```python
from build123d import *

# Parameters (mm, degrees)
PAD002_DEPTH    = 12.7
SKETCH003_W     = 152.4
SKETCH003_H     = 25.4
SKETCH003_R     = 6.35
PAD003_DEPTH    = 12.7
SKETCH006_R     = 3.175
POCKET001_DEPTH = 6.35
FILLET_R        = 12.446
SKETCH_W        = 76.2
SKETCH_H        = 50.8
SKETCH_W_2      = 73.2
SKETCH_H_2      = 47.8
PAD_DEPTH       = 1042.67
SKETCH001_W     = 76.2
SKETCH001_H     = 50.8
SKETCH001_W_2   = 73.2
SKETCH001_H_2   = 47.8
PAD001_DEPTH    = 914.4
SKETCH004_R     = 3.96875
POCKET_DEPTH    = 6.35
PAD004_DEPTH    = 1016


with BuildPart() as frameupright:
    # Sketch002 → Pad002 (new body, symmetric)
    with BuildSketch(Plane.YZ):
        Polygon((38.1, 878.1034), (38.1, 25.4), (-38.1, 25.4), (-38.1, 746.121128), align=None)
    extrude(amount=PAD002_DEPTH, both=True)

    # Sketch003 (on Face4 of Pad002) → Pad003 (join)
    with BuildSketch(Plane(origin=(0, -351.654926, 203.028066), x_dir=(0, -0.5, -0.866025), z_dir=(0, -0.866025, 0.5))):
        with Locations((-703.309852, 0)):
            Rectangle(SKETCH003_W, SKETCH003_H)
        with Locations((-754.109852, 0)):
            Circle(SKETCH003_R, mode=Mode.SUBTRACT)
        with Locations((-652.509852, 0)):
            Circle(SKETCH003_R, mode=Mode.SUBTRACT)
    extrude(amount=PAD003_DEPTH)

    # Sketch006 (on Face1 of Pad003) → Pocket001 (cut)
    with BuildSketch(Plane.ZX.offset(38.1)):
        with Locations((714.375, -0.082469)):
            Circle(SKETCH006_R)
    extrude(amount=-POCKET001_DEPTH, mode=Mode.SUBTRACT)

    # Fillet
    fillet_edges = [frameupright.edges().sort_by_distance(p)[0] for p in [
        (0, 27.101477, 884.4534),
    ]]
    fillet(fillet_edges, radius=FILLET_R)


with BuildPart() as frameupright_1:
    # Body001 placement: moved
    add(frameupright.part.moved(Location((-1029.1, 0, 0))))


with BuildPart() as frameupright001:
    # Link base: copy of FrameUpright
    add(frameupright_1.part)


with BuildPart() as frameupright001_1:
    # Link placement: moved
    add(frameupright001.part.moved(Location((2057.8, 0, 0))))


with BuildPart() as fusion:
    # Sketch → Pad (new body, symmetric)
    with BuildSketch(Plane.YZ):
        Rectangle(SKETCH_W, SKETCH_H)
        Rectangle(SKETCH_W_2, SKETCH_H_2, mode=Mode.SUBTRACT)
    extrude(amount=PAD_DEPTH, both=True)

    # Sketch001 (on DatumPlane) → Pad001 (join)
    with BuildSketch(Plane(origin=(-1079.5, -609.6, 0), x_dir=(1, 0, 0), z_dir=(0, -1, 0))):
        Rectangle(SKETCH001_W, SKETCH001_H)
        Rectangle(SKETCH001_W_2, SKETCH001_H_2, mode=Mode.SUBTRACT)
        with Locations((2159, 0)):
            Rectangle(SKETCH001_W, SKETCH001_H)
        with Locations((2159, 0)):
            Rectangle(SKETCH001_W_2, SKETCH001_H_2, mode=Mode.SUBTRACT)
    extrude(amount=-PAD001_DEPTH)

    # Sketch004 (on Face12 of Pad001) → Pocket (cut)
    with BuildSketch(Plane.YX.offset(25.4)):
        with Locations((-588.9498, -1057.275)):
            Circle(SKETCH004_R)
        with Locations((-512.7498, -1057.275)):
            Circle(SKETCH004_R)
        with Locations((-588.9498, -1101.725)):
            Circle(SKETCH004_R)
        with Locations((-512.7498, -1101.725)):
            Circle(SKETCH004_R)
        with Locations((207.9498, -1057.275)):
            Circle(SKETCH004_R)
        with Locations((207.9498, -1101.725)):
            Circle(SKETCH004_R)
        with Locations((284.1498, -1057.275)):
            Circle(SKETCH004_R)
        with Locations((284.1498, -1101.725)):
            Circle(SKETCH004_R)
    pocket = extrude(amount=-POCKET_DEPTH, mode=Mode.SUBTRACT)

    # Mirrored: Pocket across Sketch004 H_Axis
    add(pocket.mirror(Plane(origin=(0, 0, -25.4), x_dir=(0, 0, -1), z_dir=(1, 0, 0))), mode=Mode.SUBTRACT)

    # Sketch005 → Pad004 (join, symmetric)
    with BuildSketch(Plane.YZ):
        Polygon((30.1625, 38.1), (33.3375, 38.1), (33.3375, 25.4), (20.6375, 25.4), (20.6375, 28.575), (30.1625, 28.575), align=None)
    extrude(amount=PAD004_DEPTH, both=True)

    # Fusion: union FrameUpright, FrameUpright001
    add(frameupright_1.part)
    add(frameupright001_1.part)


solid = fusion.part
```
Part model, mm, in its own coordinate system. A direction names the side the tool comes from. Coordinates: 2 decimals unless noted, no trailing zeros. Order: outer loops, then holes, each group sorted by start corner. A loop starts at its lowest first (then second) coordinate and runs counter-clockwise, first axis right, second up. Notation, with made-up numbers: (9, 20.5) - (46, 20.5) arc R9 cw to (46, 30.5) - close; hole circle Ø2 at (-35.5, 77.5). An arc over 180 degrees is marked (long way). Return JSON: item names as keys, results as strings. Group by question number.
Item 1: Pin check, flat tips, straight feed: pin 1 (12.5 mm diameter, centred on x = -1057.28, y = -588.95, fed in from +Z); pin 2 (5 mm diameter, centred on x = -1029.5, z = 715.5, fed in from +Y); pin 3 (8 mm diameter, centred on y = 26.5, z = 685, fed in from -X). Stop position of each tip, or through.
Item 2: Pull direction Z, two halves, no side cores. Call faces 5 (the face through (1028.88, -13.62, 813.92)), 6 (the face through (-1080, -159, -23.9)), 7 (the face through (5, 38.1, -7)): pulls with the +Z half, pulls with the -Z half, needs draft (parallel to the pull), parting line crosses it, or undercut.
Item 3: Which spindle directions (+Z, -Z, +X, -X, +Y, -Y) get a long thin tool onto all of the face, cutting with end or side? Do faces 1 (the face through (15, -36.6, 0)), 2 (the face through (-1091, -609.6, -24.3)), 3 (the face through (1116.1, -159, 0)), 4 (the face through (-1041.4, 170, 0)). Say none if no direction does.
Item 4: Cut at A-A (z = 230). List the corners of the cut face in (x, y).
Item 5: Cut at B-B (x = -654.5). List the corners of the cut face in (y, z) (1 decimal).
Item 6: Cut at C-C (z = 813.5). List the corners of the cut face in (x, y).
Item 7: Drill centre lines: probe 1 along X at (y, z) = (34, 449); probe 2 along Z at (x, y) = (204, 34). Where is each one in solid material? Low to high. Write a range as from..to.
Check values:
{
 "1": {"pin 1": "stops at z = 25.4", "pin 2": "stops at y = 38.1", "pin 3": "stops at x = -1041.8"},
 "2": {"face 5": "pulls with the +Z half", "face 6": "undercut", "face 7": "needs draft"},
 "3": {"face 1": "none", "face 2": "+Z, -Z, +X, -X, -Y", "face 3": "+Y, -Y", "face 4": "+Z, -Z, +Y"},
 "4": {"outline": "(-1041.8, -38.1) - (-1016.4, -38.1) - (-1016.4, 38.1) - (-1041.8, 38.1) - close; (1016, -38.1) - (1041.4, -38.1) - (1041.4, 38.1) - (1016, 38.1) - close"},
 "5": {"outline": "(-38.1, -25.4) - (38.1, -25.4) - (38.1, 25.4) - (33.3, 25.4) - (33.3, 38.1) - (30.2, 38.1) - (30.2, 28.6) - (20.6, 28.6) - (20.6, 25.4) - (-38.1, 25.4) - close; hole (-36.6, -23.9) - (36.6, -23.9) - (36.6, 23.9) - (-36.6, 23.9) - close"},
 "6": {"outline": "(-1041.8, -13.86) - (-1016.4, -13.86) - (-1016.4, 38.1) - (-1041.8, 38.1) - close; (1016, -13.86) - (1041.4, -13.86) - (1041.4, 38.1) - (1016, 38.1) - close"},
 "7": {"probe 1": "x = -1041.8..-1016.4, 1016..1041.4", "probe 2": "z = -25.4..-23.9, 23.9..25.4"}
}
